Source: CAD feature listing. Evaluate the final solid. Frame: model axes, mm. Coordinates: 2 decimals unless noted, no trailing zeros. Loops run counter-clockwise (first coordinate to the right, second up) from the corner with the lowest first, then second, coordinate; pieces in that order, holes last.
Item 1: Section query C-C, the plane z = 1.45. Return the cut outline in (x, y).
Item 2: Pin query (flat end, axial travel): pin 1 Ø3 at (x, y) = (54.5, 36.5) entering from +Z; pin 2 Ø12 at (x, y) = (43.5, -16) entering from -Z; pin 3 Ø2 at (x, y) = (-54.5, -36.5) entering from -Z. Return the tip coordinate at first contact, or that it passes through.
Item 3: Line query: probe 1 along Y at (x, z) = (54.5, 2.45); probe 2 along Y at (x, z) = (30, 1.15); probe 3 along Y at (x, z) = (33, 3.4). Output: solid intervals per line, ascending.
Item 4: Section query B-B, the plane y = -20. Return the cut outline in (x, z).
Item 5: Section query A-A, the plane x = -21.5. Return the cut outline in (y, z), then the cut area to 3 significant figures.
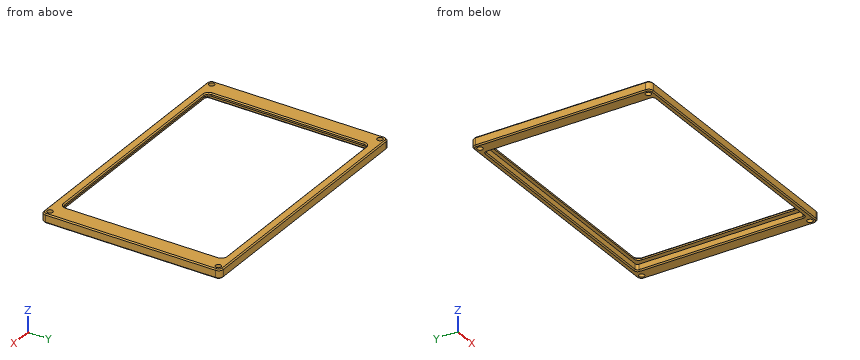
```python
from build123d import *

# Parameters (mm, degrees)
SKETCH1_W                = 113.8
SKETCH1_H                = 77.8
SKETCH1_W_2              = 98
SKETCH1_H_2              = 70
BOSS_EXTRUDE1_DEPTH      = 4
M2_CLEARANCE_HOLE1_D     = 2.4
M2_CLEARANCE_HOLE1_DEPTH = 4
FILLET1_R                = 2
FILLET2_R                = 2
SKETCH5_W                = 102.2
SKETCH5_H                = 73
CUT_EXTRUDE2_DEPTH       = 2.8
FILLET5_R                = 1
CHAMFER1_SIZE            = 0.5


with BuildPart() as part:
    # Sketch1 → Boss-Extrude1 (new body)
    with BuildSketch(Plane.XY):
        Rectangle(SKETCH1_W, SKETCH1_H)
        Rectangle(SKETCH1_W_2, SKETCH1_H_2, mode=Mode.SUBTRACT)
    extrude(amount=BOSS_EXTRUDE1_DEPTH)

    # M2 Clearance Hole1
    with Locations(Plane.XY.offset(4)):
        with Locations((0, 0), (54.5, 36.5), (-54.5, -36.5), (-54.5, 36.5), (54.5, -36.5)):
            Hole(M2_CLEARANCE_HOLE1_D / 2, depth=M2_CLEARANCE_HOLE1_DEPTH)

    # Fillet1
    fillet1_edges = [part.edges().sort_by_distance(p)[0] for p in [
        (56.9, -38.9, 2),
        (-56.9, -38.9, 2),
        (-56.9, 38.9, 2),
        (56.9, 38.9, 2),
    ]]
    fillet(fillet1_edges, radius=FILLET1_R)

    # Fillet2
    fillet2_edges = [part.edges().sort_by_distance(p)[0] for p in [
        (49, -35, 2),
        (49, 35, 2),
        (-49, 35, 2),
        (-49, -35, 2),
    ]]
    fillet(fillet2_edges, radius=FILLET2_R)

    # Sketch5 → Cut-Extrude2 (cut)
    with BuildSketch(Plane(origin=(0, 0, 0), x_dir=(-1, 0, 0), z_dir=(0, 0, -1))):
        Rectangle(SKETCH5_W, SKETCH5_H)
    extrude(amount=-CUT_EXTRUDE2_DEPTH, mode=Mode.SUBTRACT)

    # Fillet5
    fillet5_edges = [part.edges().sort_by_distance(p)[0] for p in [
        (-51.1, 36.5, 1.4),
        (-51.1, -36.5, 1.4),
        (51.1, -36.5, 1.4),
        (51.1, 36.5, 1.4),
    ]]
    fillet(fillet5_edges, radius=FILLET5_R)

    # Chamfer1
    chamfer1_edges = [part.edges().sort_by_distance(p)[0] for p in [
        (0, -36.5, 0),
        (51.1, 0, 0),
        (0, 36.5, 0),
        (-51.1, 0, 0),
        (50.807106781, -36.207106781, 0),
        (-50.807106781, 36.207106781, 0),
        (-50.807106781, -36.207106781, 0),
        (50.807106781, 36.207106781, 0),
        (56.9, 0, 0),
        (56.9, 0, 4),
        (0, -38.9, 0),
        (-56.9, 0, 0),
        (0, 38.9, 0),
        (-56.314213562, 38.314213562, 0),
        (56.314213562, 38.314213562, 0),
        (-56.314213562, -38.314213562, 0),
        (56.314213562, -38.314213562, 0),
        (0, -38.9, 4),
        (0, 38.9, 4),
        (-56.9, 0, 4),
        (-56.314213562, 38.314213562, 4),
        (56.314213562, 38.314213562, 4),
        (-56.314213562, -38.314213562, 4),
        (56.314213562, -38.314213562, 4),
        (49, 0, 4),
        (0, 35, 4),
        (-49, 0, 4),
        (0, -35, 4),
        (48.414213562, 34.414213562, 4),
        (-48.414213562, -34.414213562, 4),
        (48.414213562, -34.414213562, 4),
        (-48.414213562, 34.414213562, 4),
    ]]
    chamfer(chamfer1_edges, length=CHAMFER1_SIZE)


solid = part.part
```
Verdict:
1. outline: (-56.9, -36.9) arc R2 ccw to (-54.9, -38.9) - (54.9, -38.9) arc R2 ccw to (56.9, -36.9) - (56.9, 36.9) arc R2 ccw to (54.9, 38.9) - (-54.9, 38.9) arc R2 ccw to (-56.9, 36.9) - close; hole circle Ø2.4 at (-54.5, -36.5); hole circle Ø2.4 at (-54.5, 36.5); hole (-51.1, -35.5) arc R1 ccw to (-50.1, -36.5) - (50.1, -36.5) arc R1 ccw to (51.1, -35.5) - (51.1, 35.5) arc R1 ccw to (50.1, 36.5) - (-50.1, 36.5) arc R1 ccw to (-51.1, 35.5) - close; hole circle Ø2.4 at (54.5, -36.5); hole circle Ø2.4 at (54.5, 36.5)
2. pin 1: stops at z = 4
2. pin 2: stops at z = 2.8
2. pin 3: passes through
3. probe 1: y = -38.9 to -37.7, -35.3 to 35.3, 37.7 to 38.9
3. probe 2: y = -38.9 to -36.5, 36.5 to 38.9
3. probe 3: y = -38.9 to -35, 35 to 38.9
4. outline: (-56.9, 0.5) - (-56.4, 0) - (-51.6, 0) - (-51.1, 0.5) - (-51.1, 2.8) - (-49, 2.8) - (-49, 3.5) - (-49.5, 4) - (-56.4, 4) - (-56.9, 3.5) - close; (49, 2.8) - (51.1, 2.8) - (51.1, 0.5) - (51.6, 0) - (56.4, 0) - (56.9, 0.5) - (56.9, 3.5) - (56.4, 4) - (49.5, 4) - (49, 3.5) - close
5. outline: (-38.9, 0.5) - (-38.4, 0) - (-37, 0) - (-36.5, 0.5) - (-36.5, 2.8) - (-35, 2.8) - (-35, 3.5) - (-35.5, 4) - (-38.4, 4) - (-38.9, 3.5) - close; (35, 2.8) - (36.5, 2.8) - (36.5, 0.5) - (37, 0) - (38.4, 0) - (38.9, 0.5) - (38.9, 3.5) - (38.4, 4) - (35.5, 4) - (35, 3.5) - close
5. area: 21.8 mm2
